For this review, take the finished solid that the model builds, in its own axes (mm). Round coordinates to 2 decimals unless told otherwise and drop trailing zeros. Order: outer loops, then holes, each group sorted by start corner. A loop starts at its lowest first (then second) coordinate and runs counter-clockwise, first axis right, second up. Notation, with made-up numbers: M 55.5,46 L 90.5,46 A20 ccw 90.5,74 Z; hole C 24,62.5 d3. An arc over 180 degrees is marked long. Use a Markdown table: item, result.
from build123d import *

# Parameters (mm, degrees)
PAD_DEPTH = 19
FILLET_R  = 30


with BuildPart() as part:
    # Sketch001 → Pad (new body)
    with BuildSketch(Plane.XZ):
        Polygon((-39.633348, -30.069131), (-39.633348, 139.930869), (114.876213, 153.448704), (227.584428, 463.11198), (101.724005, 535.777529), (158.157329, 690.826811), (435.366652, 589.930869), (435.366652, -30.069131), align=None)
    extrude(amount=-PAD_DEPTH)

    # Fillet
    fillet_edges = [part.edges().sort_by_distance(p)[0] for p in [
        (-39.633348, 9.5, -30.069131),
        (-39.633348, 9.5, 139.930869),
        (101.724005, 9.5, 535.777529),
        (158.157329, 9.5, 690.826811),
        (435.366652, 9.5, 589.930869),
        (227.584428, 9.5, 463.11198),
        (114.876213, 9.5, 153.448704),
    ]]
    fillet(fillet_edges, radius=FILLET_R)


solid = part.part
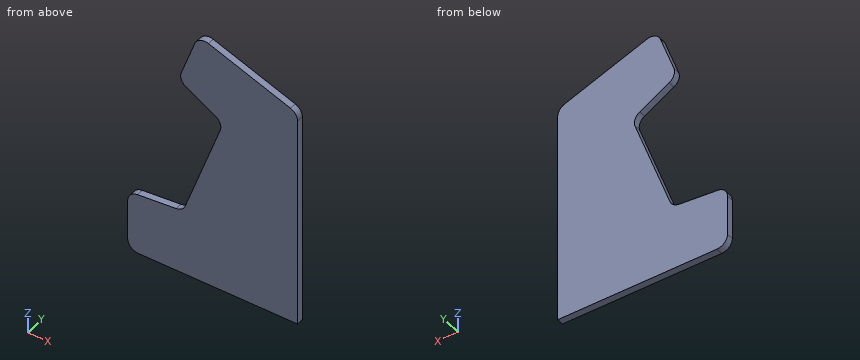
Q1. Add section A-A (y = 15.5). Write out the cut boundary in (x, z), then the cut area to 3 significant figures.
Determined:
| item | result |
|---|---|
| outline | M -39.63,-0.07 A30 ccw -9.63,-30.07 L 435.37,-30.07 L 435.37,568.92 A30 ccw 415.63,597.12 L 186.35,680.57 A30 ccw 147.9,662.64 L 110.33,559.43 A30 ccw 123.52,523.19 L 205.78,475.7 A30 cw 218.97,439.46 L 121.41,171.41 A30 cw 95.84,151.78 L -12.25,142.33 A30 ccw -39.63,112.44 Z |
| area | 220,000 mm^2 |
Q2. Add section B-B (x = 9). Write out the cut boundary in (y, z).
Determined:
| item | result |
|---|---|
| outline | M 0,-30.07 L 19,-30.07 L 19,144.19 L 0,144.19 Z |
Q3. Clearance check with flat-ended pins moving along their axes: pin 1 (1.5 mm diameter, centred on x = 340, y = 10, fed in from +Z); pin 2 (1.5 mm diameter, centred on y = 8, z = 281.5, fed in from -X). State where each tip first meets the part, or that it passes through.
Determined:
| item | result |
|---|---|
| pin 1 | stops at z = 624.91 |
| pin 2 | stops at x = 161.21 |
Q4. Add section C-C (z = 291). Write out the cut boundary in (x, y), then the cut area to 3 significant figures.
Determined:
| item | result |
|---|---|
| outline | M 164.94,0 L 435.37,0 L 435.37,19 L 164.94,19 Z |
| area | 5,140 mm^2 |
Q5. Wall thickness on line 1 along X through (y, z) = (5.5, 549.5); line 2 along Z through (x, y) = (50, 1.5); line 3 along Z through (x, y) = (-3.5, 6.5): over which ranges is each line inside the solid? List them lowest first. Write a range as [from, to].
Determined:
| item | result |
|---|---|
| line 1 | x = [108.53, 435.37] |
| line 2 | z = [-30.07, 147.77] |
| line 3 | z = [-30.07, 143.09] |
